For this review, take the finished solid that the model builds, in its own axes (mm). Face numbers are marked on the shaded views. Give positions to 0.01 mm unless a question says otherwise; leave off trailing zeros. Loops run counter-clockwise (first coordinate to the right, second up) from the corner with the lowest first, then second, coordinate; pieces in that order, holes last. Notation, with made-up numbers: M 62,-17.5 L 82,-17.5 A31 cw 82,19.5 Z; hole C 77.25,62 d5. An arc over 180 degrees is marked long. Use CSV: the item, a comma, the result in double quotes. Start each with the question number.
1. The part is to be moulded in two halves that separate along Y. For the marked faces 1, 2 and 3, say which applies: pulls with the +Y half, pulls with the -Y half, needs draft (parallel to the pull), parting line crosses it, or undercut.
2. Take a section at A-A, the plane x = 0. Write out the cut boundary in (y, z), and give its area (3 significant figures).
3. To check wall thickness, follow line 1 (Y direction, x = 0, z = 2); line 2 (Y direction, x = -1.75, z = 3.75). State the ranges of each line that lie inside material, in increasing order. Write a range as [from, to].
4. Take a section at B-B, the plane y = -15. Write out the cut boundary in (x, z) (3 decimals), and give its area (3 significant figures).
5. Insertion check: P1, Ø3.5, axis at x = 0, y = -15, coming from the -Z side. The pin has a flat end and moves straight along its axis. Give the tip position at first contact, or say it passes through.
6. Take a section at C-C, the plane z = -0.5. Write out the cut boundary in (x, y) (3 decimals).
from build123d import *

# Parameters (mm, degrees)
F0_W     = 19.05
F0_H     = 12.7
F1_DEPTH = 25
F3_D     = 4.5


with BuildPart() as f1:
    # F0 (on Front) → F1 (new body, symmetric)
    with BuildSketch(Plane.XZ):
        Rectangle(F0_W, F0_H)
    extrude(amount=F1_DEPTH, both=True)

    # F3 (through all)
    with Locations(Plane.XY.offset(6.35)):
        with Locations((0, 15), (0, -15)):
            Hole(F3_D / 2)


solid = f1.part
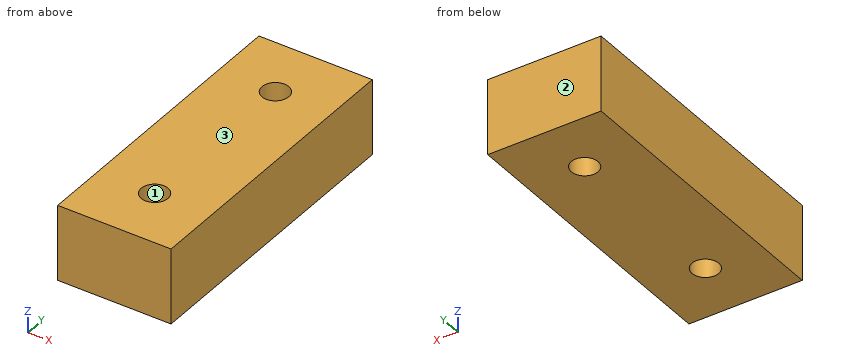
Result set:
1,face 1,"undercut"
1,face 2,"pulls with the +Y half"
1,face 3,"needs draft"
2,outline,"M -25,-6.35 L -17.25,-6.35 L -17.25,6.35 L -25,6.35 Z; M -12.75,-6.35 L 12.75,-6.35 L 12.75,6.35 L -12.75,6.35 Z; M 17.25,-6.35 L 25,-6.35 L 25,6.35 L 17.25,6.35 Z"
2,area,"521 mm2"
3,line 1,"[-25, -17.25], [-12.75, 12.75], [17.25, 25]"
3,line 2,"[-25, -16.41], [-13.59, 13.59], [16.41, 25]"
4,outline,"M -9.525,-6.35 L -2.25,-6.35 L -2.25,6.35 L -9.525,6.35 Z; M 2.25,-6.35 L 9.525,-6.35 L 9.525,6.35 L 2.25,6.35 Z"
4,area,"185 mm2"
5,P1,"through"
6,outline,"M -9.525,-25 L 9.525,-25 L 9.525,25 L -9.525,25 Z; hole C 0,-15 d4.5; hole C 0,15 d4.5"
